Model file for the job. Use its own axes, mm. Face numbers are marked on the shaded views. Round coordinates to 2 decimals unless told otherwise and drop trailing zeros. Loops run counter-clockwise (first coordinate to the right, second up) from the corner with the lowest first, then second, coordinate; pieces in that order, holes last. Notation, with made-up numbers: (-3, 81.25) -> (28, 81.25) arc R14 ccw to (28, 106.25) -> close; hole circle Ø11 at (13.5, 25). An arc over 180 degrees is marked (long way). Use a Markdown table: item, result.
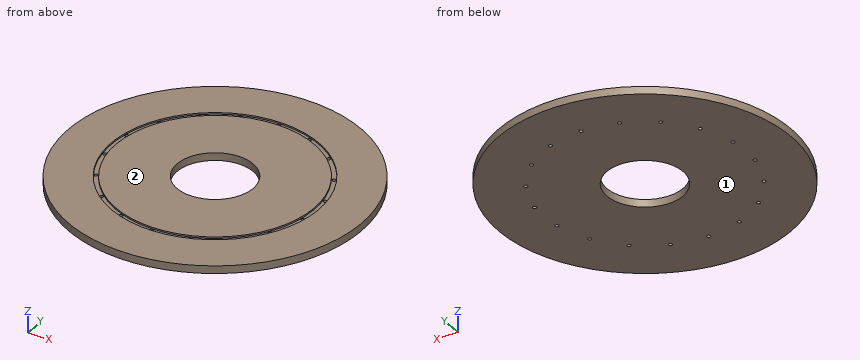
Autodesk Inventor part; units mm, degrees
ref_plane "YZ Plane" through (0, 0, 0) normal (1, 0, 0) x (0, 1, 0)
ref_plane "XZ Plane" through (0, 0, 0) normal (0, 1, 0) x (-1, 0, 0)
ref_plane "XY Plane" through (0, 0, 0) normal (0, 0, 1) x (1, 0, 0)
sketch "Boceto1" plane through (0, 0, 0) normal (0, 0, 1) x (1, 0, 0)
  circle A0 centre (0, 0) radius 125
  circle A1 centre (0, 0) radius 480
  dimension "d0" = 960
  dimension "d1" = 250
extrude "Extrusión1" add sketch "Boceto1" against normal blind 25
sketch "Boceto2" plane through (0, 0, 0) normal (0, 0, 1) x (1, 0, 0)
  circle A0 centre (0, 0) radius 340
  circle A1 centre (0, 0) radius 325
  dimension "d4" = 680
  dimension "d5" = 650
extrude "Extrusión2" cut sketch "Boceto2" against normal blind 5
sketch "Boceto3" plane through (0, 0, 0) normal (0, 0, 1) x (1, 0, 0)
  circle A0 centre (0, 0) radius 332.5 construction
  circle A1 centre (0, 332.5) radius 6
  circle A2 centre (-113.7217, 312.4478) radius 6
  circle A3 centre (-213.7269, 254.7098) radius 6
  circle A4 centre (-287.9534, 166.25) radius 6
  circle A5 centre (-327.4486, 57.738) radius 6
  circle A6 centre (-327.4486, -57.738) radius 6
  circle A7 centre (-287.9534, -166.25) radius 6
  circle A8 centre (-213.7269, -254.7098) radius 6
  circle A9 centre (-113.7217, -312.4478) radius 6
  circle A10 centre (0, -332.5) radius 6
  circle A11 centre (113.7217, -312.4478) radius 6
  circle A12 centre (213.7269, -254.7098) radius 6
  circle A13 centre (287.9534, -166.25) radius 6
  circle A14 centre (327.4486, -57.738) radius 6
  circle A15 centre (327.4486, 57.738) radius 6
  circle A16 centre (287.9534, 166.25) radius 6
  circle A17 centre (213.7269, 254.7098) radius 6
  circle A18 centre (113.7217, 312.4478) radius 6
  dimension "d8" = 665
  dimension "d9" = 12
  dimension "d12" = 360
extrude "Extrusión3" cut sketch "Boceto3" against normal up to next
properties part number "Brida_2 (flange_2)"
Q1. Band-saw the part on B-B, the plane y = 186. Give the cut face in (x, z), plus the area to 3 significant figures.
Results list:
| item | result |
|---|---|
| outline | (-442.5, -25) -> (442.5, -25) -> (442.5, 0) -> (284.61, 0) -> (284.61, -5) -> (266.51, -5) -> (266.51, 0) -> (-266.51, 0) -> (-266.51, -5) -> (-284.61, -5) -> (-284.61, 0) -> (-442.5, 0) -> close |
| area | 21,900 mm² |
Q2. Flat gauge pins, fed straight in: pin 1 (12 mm diameter, centred on x = 209.5, z = -17, fed in from +Y); pin 2 (5 mm diameter, centred on y = 229.5, z = -18, fed in from -X); pin 3 (6 mm diameter, centred on y = -288, z = -14, fed in from +X). Where does each tip first touch, or does it go through?
Results list:
| item | result |
|---|---|
| pin 1 | stops at y = 434.73 |
| pin 2 | stops at x = -422.93 |
| pin 3 | stops at x = 386.23 |
Q3. Band-saw the part on A-A, the plane z = -11.5. Give the number of separate pieces and of enclosed holes in the cut face, plus the area to 3 significant figures.
Results list:
| item | result |
|---|---|
| separate pieces | 1 |
| enclosed holes | 19 |
| area | 673,000 mm² |
Q4. Band-saw the part on C-C, the plane y = 379. Give the cut face in (x, z), plus the area to 3 significant figures.
Results list:
| item | result |
|---|---|
| outline | (-294.55, -25) -> (294.55, -25) -> (294.55, 0) -> (-294.55, 0) -> close |
| area | 14,700 mm² |
Q5. Drill centre lines: L1, parallel to Y at x = 290, z = -10.5; L2, parallel to Y at x = -212.5, z = -15; L3, parallel to X at y = 31, z = -1.5 (3 decimals). Where is each one in solid material? Low to high. Write a range as from..to.
Results list:
| item | result |
|---|---|
| L1 | y = -382.49..-171.89, -160.61..160.61, 171.89..382.49 |
| L2 | y = -430.4..-260.58, -248.84..248.84, 260.58..430.4 |
| L3 | x = -478.998..-338.584, -323.518..-121.095, 121.095..323.518, 338.584..478.998 |
Q6. Band-saw the part on D-D, the plane y = -395. Give the cut face in (x, z).
Results list:
| item | result |
|---|---|
| outline | (-272.72, -25) -> (272.72, -25) -> (272.72, 0) -> (-272.72, 0) -> close |
Q7. Pull direction Z, two halves, no side cores. Call the marked faces 1 and 2: released by +Z, released by -Z, zero draft, split by the parting line, or undercut.
Results list:
| item | result |
|---|---|
| face 1 | released by -Z |
| face 2 | released by +Z |
